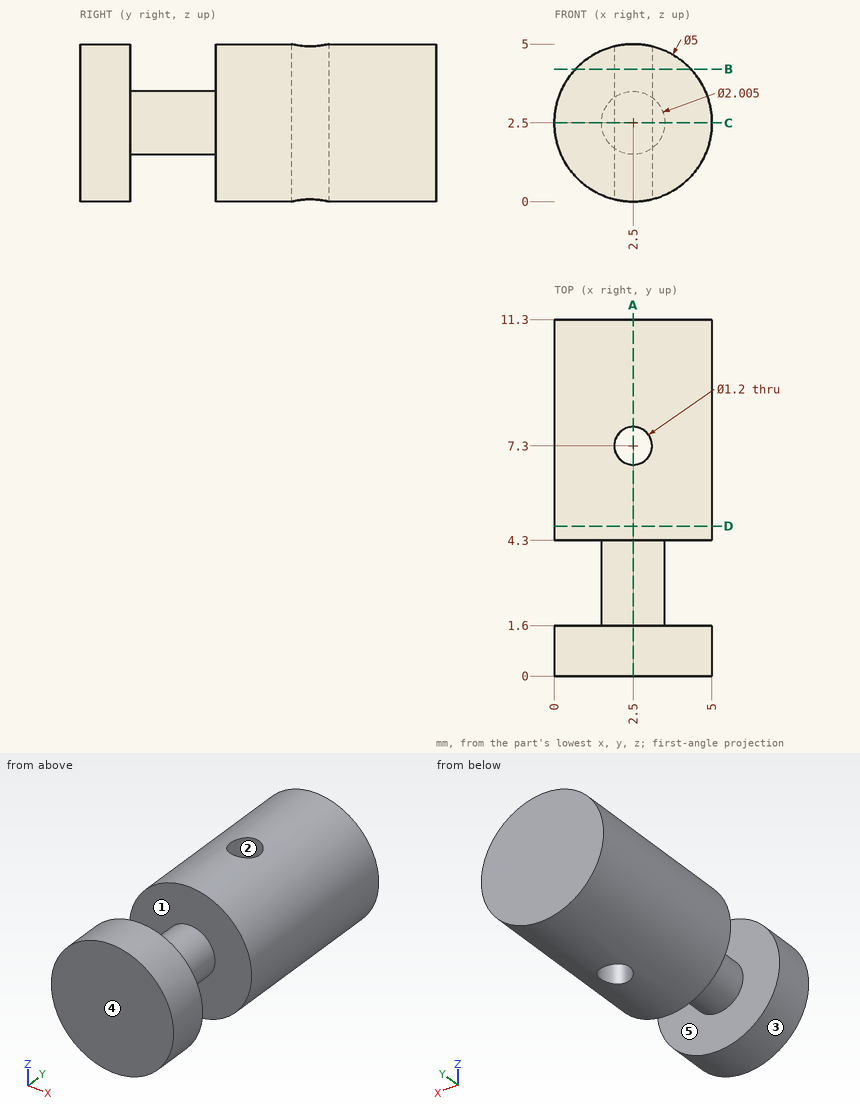
Can you work these out from the drawing? Everything is in mm from the part's minimum corner. A direction names the side the tool comes from. Coordinates: 2 decimals unless noted, no trailing zeros. Order: outer loops, then holes, each group sorted by start corner. A loop starts at its lowest first (then second) coordinate and runs counter-clockwise, first axis right, second up. Notation, with made-up numbers: (3.5, 34) -> (21.5, 34) arc R28 cw to (21.5, 62) -> close; hole circle Ø6 at (51.25, -28). An arc over 180 degrees is marked (long way). Return JSON: item names as keys, results as strings.
1) If we section it at D-D on y = 4.75: List the corners of the cut face in (x, z) for me.
Conclusion:
{"outline": "circle Ø5 at (2.5, 2.5)"}
2) If we section it at A-A on x = 2.5: List the corners of the cut face in (y, z) for me.
Conclusion:
{"outline": "(0, 0) -> (1.6, 0) -> (1.6, 1.5) -> (4.3, 1.5) -> (4.3, 0) -> (6.7, 0) -> (6.7, 5) -> (4.3, 5) -> (4.3, 3.5) -> (1.6, 3.5) -> (1.6, 5) -> (0, 5) -> close; (7.9, 0) -> (11.3, 0) -> (11.3, 5) -> (7.9, 5) -> close"}
3) I'm going to push flat-ended pins straight in: P1, Ø3, axis at x = 1.5, y = 6, coming from the +Z side; P2, Ø1.5, axis at y = 7.5, z = 1.5, coming from the +X side. Where does each tip first touch, or does it pass through?
Conclusion:
{"P1": "stops at z = 5", "P2": "stops at x = 4.99"}
4) If we section it at C-C on z = 2.5: List the corners of the cut face in (x, y) for me.
Conclusion:
{"outline": "(0, 0) -> (5, 0) -> (5, 1.6) -> (3.5, 1.6) -> (3.5, 4.3) -> (5, 4.3) -> (5, 11.3) -> (0, 11.3) -> (0, 4.3) -> (1.5, 4.3) -> (1.5, 1.6) -> (0, 1.6) -> close; hole circle Ø1.2 at (2.5, 7.3)"}
5) If we section it at B-B on z = 4.2: List the corners of the cut face in (x, y) for me, plus the area to 3 significant figures.
Conclusion:
{"outline": "(0.67, 0) -> (4.33, 0) -> (4.33, 1.6) -> (0.67, 1.6) -> close; (0.67, 4.3) -> (4.33, 4.3) -> (4.33, 11.3) -> (0.67, 11.3) -> close; hole circle Ø1.2 at (2.5, 7.3)", "area": "30.4 mm²"}
6) On a 3-axis mill with a long thin cutter (end or side, diameter ignored), from which of +Z, -Z, +X, -X, +Y, -Y can I reach the whole of each face in a straight line? I mean the marked faces 1 and 2. Say none if no direction works.
Conclusion:
{"face 1": "none", "face 2": "+Z, -Z"}
7) If I drill on probe 1 along X at (y, z) = (7.3, 2.5); probe 2 along Y at (x, z) = (0.6, 3.15); probe 3 along Y at (x, z) = (2.35, 4), over which ranges is the centre line in solid material (lowest first)?
Conclusion:
{"probe 1": "x = 0 to 1.9, 3.1 to 5", "probe 2": "y = 0 to 1.6, 4.3 to 11.3", "probe 3": "y = 0 to 1.6, 4.3 to 6.72, 7.88 to 11.3"}
8) Thinking about a two-plate mould opening in Y: for the marked faces 3, 4 and 5, which applies, +Y half, -Y half, draft (parallel to the pull), parting line (faces both ways), or undercut?
Conclusion:
{"face 3": "draft", "face 4": "-Y half", "face 5": "undercut"}
